```python
from build123d import *

# Parameters (mm, degrees)
SKETCH_1_W      = 31
SKETCH_1_H      = 42
SKETCH_1_R      = 1.5
EXTRUDE_1_DEPTH = 1
SKETCH_2_W      = 5
SKETCH_2_H      = 5
EXTRUDE_2_DEPTH = 3
SKETCH_3_W      = 3
SKETCH_3_H      = 4.5
SKETCH_3_W_2    = 2.541472094
SKETCH_3_H_2    = 0.485869665
EXTRUDE_3_DEPTH = 1
SKETCH_4_W      = 3
SKETCH_4_H      = 1
EXTRUDE_4_DEPTH = 1
SKETCH_5_W      = 1.5
SKETCH_5_H      = 5
EXTRUDE_5_DEPTH = 2


with BuildPart() as part:
    # 草圖1 → 填料-伸長1 (new body)
    with BuildSketch(Plane(origin=(0, 0, 0), x_dir=(1, 0, 0), z_dir=(0, 1, 0))):
        with Locations((15.5, 21)):
            Rectangle(SKETCH_1_W, SKETCH_1_H)
        with Locations((5, 21)):
            Circle(SKETCH_1_R, mode=Mode.SUBTRACT)
    extrude(amount=EXTRUDE_1_DEPTH)

    # 草圖2 → 填料-伸長2 (add)
    with BuildSketch(Plane(origin=(0, 1, 0), x_dir=(1, 0, 0), z_dir=(0, 1, 0))):
        with Locations((12.5, 2.5)):
            Rectangle(SKETCH_2_W, SKETCH_2_H)
    extrude(amount=EXTRUDE_2_DEPTH)

    # 草圖3 → 填料-伸長3 (add)
    with BuildSketch(Plane(origin=(0, 1, 0), x_dir=(1, 0, 0), z_dir=(0, 1, 0))):
        with Locations((12.476364023, 9.25)):
            Rectangle(SKETCH_3_W, SKETCH_3_H)
        with Locations((19.871516351, 12.595108575)):
            Rectangle(SKETCH_3_W_2, SKETCH_3_H_2)
        with Locations((19.871516351, 10.595108575)):
            Rectangle(SKETCH_3_W_2, SKETCH_3_H_2)
        with Locations((19.871516351, 8.595108574)):
            Rectangle(SKETCH_3_W_2, SKETCH_3_H_2)
        with Locations((19.871516351, 6.595108575)):
            Rectangle(SKETCH_3_W_2, SKETCH_3_H_2)
        with Locations((19.871516351, 4.595108575)):
            Rectangle(SKETCH_3_W_2, SKETCH_3_H_2)
        with Locations((19.871516351, 2.595108575)):
            Rectangle(SKETCH_3_W_2, SKETCH_3_H_2)
    extrude(amount=EXTRUDE_3_DEPTH)

    # 草圖4 → 填料-伸長4 (add)
    with BuildSketch(Plane(origin=(0, 1, 0), x_dir=(1, 0, 0), z_dir=(0, 1, 0))):
        with Locations((5, 25)):
            Rectangle(SKETCH_4_W, SKETCH_4_H)
        with Locations((5, 17)):
            Rectangle(SKETCH_4_W, SKETCH_4_H)
    extrude(amount=EXTRUDE_4_DEPTH)

    # 草圖5 → 填料-伸長5 (add)
    with BuildSketch(Plane(origin=(0, 1, 0), x_dir=(1, 0, 0), z_dir=(0, 1, 0))):
        with Locations((0.75, 6.944626386)):
            Rectangle(SKETCH_5_W, SKETCH_5_H)
    extrude(amount=EXTRUDE_5_DEPTH)


solid = part.part
```
For this review, take the finished solid that the model builds, in its own axes (mm). A direction names the side the tool comes from. Give positions to 0.01 mm unless a question says otherwise; leave off trailing zeros. Write each loop counter-clockwise with the first axis right and the second up, starting at its lowest first coordinate (ties: lowest second). Pieces come first, ordered by that corner, then holes. Notation, with made-up numbers: M 45.25,7.25 L 71.25,7.25 A19 cw 71.25,42.25 Z; hole C 74,-2 d2. An arc over 180 degrees is marked long. Answer as CSV lines item,"result".
1. For pin 1 (0.5 mm diameter, centred on x = 5.5, y = 1.5, fed in from +Z); pin 2 (2 mm diameter, centred on x = 22, z = -24.5, fed in from +Y); pin 3 (1 mm diameter, centred on y = 2.5, z = -37, fed in from +X); pin 4 (0.8 mm diameter, centred on x = 5, z = -25, fed in from +Y), all flat-tipped, find the tip position at first contact; note any pin that passes through.
Findings:
pin 1,"stops at z = -16.5"
pin 2,"stops at y = 1"
pin 3,"passes through"
pin 4,"stops at y = 2"
2. Consider section A-A, the plane z = -21. Write out the cut boundary in (x, y).
Findings:
outline,"M 0,0 L 3.5,0 L 3.5,1 L 0,1 Z; M 6.5,0 L 31,0 L 31,1 L 6.5,1 Z"
3. For faces 1 (the flat face through (12, 2, -5)), 2 (the flat face through (19.9, 1.5, -2.352)), 3 (the flat face through (6.5, 1.5, -25)), 4 (the flat face through (19.9, 1.5, -12.838)), 5 (the flat face through (13.976, 1.5, -9.2)), list the 3-axis set-ups (+Z, -Z, +X, -X, +Y, -Y) from which the entire face can be reached by the end or side of a thin tool; tool diameter is ignored.
Findings:
face 1,"+X, +Y"
face 2,"+Z, +X, +Y"
face 3,"+Z, -Z, +X, +Y"
face 4,"-Z, +X, -X, +Y"
face 5,"-Z, +Y"
4. Consider section B-B, the plane x = 5. Write out the cut boundary in (y, z).
Findings:
outline,"M 0,-42 L 1,-42 L 1,-25.5 L 2,-25.5 L 2,-24.5 L 1,-24.5 L 1,-22.5 L 0,-22.5 Z; M 0,-19.5 L 1,-19.5 L 1,-17.5 L 2,-17.5 L 2,-16.5 L 1,-16.5 L 1,0 L 0,0 Z"
5. Wall thickness on line 1 (X direction, y = 0.4, z = -21); line 2 (Z direction, x = 5, y = 0.65); line 3 (X direction, y = 3.7, z = -2.5): over which ranges is each line inside the solid? List them lowest first.
Findings:
line 1,"x = 0 to 3.5, 6.5 to 31"
line 2,"z = -42 to -22.5, -19.5 to 0"
line 3,"x = 10 to 15"
6. Consider section C-C, the plane x = 11.5. Write out the cut boundary in (y, z), then the cut area to 3 significant figures.
Findings:
outline,"M 0,-42 L 1,-42 L 1,-11.5 L 2,-11.5 L 2,-7 L 1,-7 L 1,-5 L 4,-5 L 4,0 L 0,0 Z"
area,"61.5 mm2"
7. Consider section D-D, the plane x = 23.5. Write out the cut boundary in (y, z), then the cut area to 3 significant figures.
Findings:
outline,"M 0,-42 L 1,-42 L 1,0 L 0,0 Z"
area,"42.0 mm2"
8. Draft analysis for pull direction Z (two halves, no side actions). For faces 6 (the flat face through (1, 2, -4.445)), 7 (the flat face through (10.976, 1.5, -9.2)), 8 (the flat face through (5, 1.5, -25.5)), 9 (the flat face through (19.9, 1.5, -6.352)), state which applies: +Z half, -Z half, draft (parallel to the pull), parting line (faces both ways), or undercut.
Findings:
face 6,"+Z half"
face 7,"draft"
face 8,"-Z half"
face 9,"undercut"
